from build123d import *

# Parameters (mm, degrees)
SKETCH1_R           = 1.5
BOSS_EXTRUDE1_DEPTH = 2
FILLET1_R           = 2


with BuildPart() as part:
    # Sketch1 → Boss-Extrude1 (new body)
    with BuildSketch(Plane(origin=(0, 0, 0), x_dir=(1, 0, 0), z_dir=(0, 1, 0))):
        Polygon((-18, 18), (18, 18), (18, -18), (8, -18), (8, -34), (-8, -34), (-8, -18), (-18, -18), align=None)
        with Locations(Location((-15, 15, 0), (0, 0, 270))):
            Circle(SKETCH1_R, mode=Mode.SUBTRACT)
        with Locations(Location((15, 15, 0), (0, 0, 90))):
            Circle(SKETCH1_R, mode=Mode.SUBTRACT)
        with Locations(Location((15, -15, 0), (0, 0, 270))):
            Circle(SKETCH1_R, mode=Mode.SUBTRACT)
        with Locations(Location((-15, -15, 0), (0, 0, 90))):
            Circle(SKETCH1_R, mode=Mode.SUBTRACT)
    extrude(amount=BOSS_EXTRUDE1_DEPTH)

    # Fillet1
    fillet1_edges = [part.edges().sort_by_distance(p)[0] for p in [
        (8, 1, 18),
        (8, 1, 34),
        (-8, 1, 34),
        (-8, 1, 18),
        (-18, 1, 18),
        (-18, 1, -18),
        (18, 1, -18),
        (18, 1, 18),
    ]]
    fillet(fillet1_edges, radius=FILLET1_R)


solid = part.part
The model under review builds one solid part; all positions refer to its coordinate system, in mm. A direction names the side the tool comes from. Coordinates: 2 decimals unless noted, no trailing zeros. Loops run counter-clockwise (first coordinate to the right, second up) from the corner with the lowest first, then second, coordinate; pieces in that order, holes last. Notation, with made-up numbers: (-12, 45) -> (7, 45) arc R23 cw to (7, 54) -> close; hole circle Ø4 at (37.25, 88.5). An arc over 180 degrees is marked (long way). Use a Markdown table: item, result. Add a question column.
1. Machinability: for faces 1 (the face through (-8, 1, 26)), 2 (the face through (14.93, 0.99, -13.5)), 3 (the face through (8, 1, 26)), which of the approach directions +Z, -Z, +X, -X, +Y, -Y give a long, thin tool a straight path to every point of the face, cutting with its end or side? Answer none if there is none.
2. Add section D-D on z = 24. Write out the cut boundary in (x, y), plus the area to 3 significant figures.
3. Add section A-A on z = -15. Write out the cut boundary in (x, y), plus the area to 3 significant figures.
4. Add section C-C on y = 1.55. Write out the cut boundary in (x, z), plus the area to 3 significant figures.
5. Add section B-B on x = -15. Write out the cut boundary in (y, z).
6. To check wall thickness, follow line 1 (X direction, y = 1, z = -15); line 2 (Z direction, x = 15.5, y = 1.8); line 3 (X direction, y = 0.4, z = 31.5). State the ranges of each line that lie inside material, in increasing order.
7. Draft analysis for pull direction Z (two halves, no side actions). For faces 4 (the face through (13, 1, 18)), 5 (the face through (15.07, 0.99, 13.5)), 6 (the face through (0, 0, 2)), state which applies: pulls with the +Z half, pulls with the -Z half, needs draft (parallel to the pull), parting line crosses it, or undercut.
8. Clearance check with flat-ended pins moving along their axes: pin 1 Ø0.6 at (y, z) = (1.5, 29) entering from -X; pin 2 Ø2.5 at (x, z) = (15, -15) entering from -Y; pin 3 Ø1 at (y, z) = (1.5, 26) entering from +X. State where each tip first meets the part, or that it passes through.
Returned:
| question | item | result |
|---|---|---|
| 1 | face 1 | +Z, -X, +Y, -Y |
| 1 | face 2 | +Y, -Y |
| 1 | face 3 | +Z, +X, +Y, -Y |
| 2 | outline | (-8, 0) -> (8, 0) -> (8, 2) -> (-8, 2) -> close |
| 2 | area | 32.0 mm² |
| 3 | outline | (-18, 0) -> (-16.5, 0) -> (-16.5, 2) -> (-18, 2) -> close; (-13.5, 0) -> (13.5, 0) -> (13.5, 2) -> (-13.5, 2) -> close; (16.5, 0) -> (18, 0) -> (18, 2) -> (16.5, 2) -> close |
| 3 | area | 60.0 mm² |
| 4 | outline | (-18, -16) arc R2 ccw to (-16, -18) -> (16, -18) arc R2 ccw to (18, -16) -> (18, 16) arc R2 ccw to (16, 18) -> (10, 18) arc R2 cw to (8, 20) -> (8, 32) arc R2 ccw to (6, 34) -> (-6, 34) arc R2 ccw to (-8, 32) -> (-8, 20) arc R2 cw to (-10, 18) -> (-16, 18) arc R2 ccw to (-18, 16) -> close; hole circle Ø3 at (-15, -15); hole circle Ø3 at (-15, 15); hole circle Ø3 at (15, -15); hole circle Ø3 at (15, 15) |
| 4 | area | 1,520 mm² |
| 5 | outline | (0, -18) -> (2, -18) -> (2, -16.5) -> (0, -16.5) -> close; (0, -13.5) -> (2, -13.5) -> (2, 13.5) -> (0, 13.5) -> close; (0, 16.5) -> (2, 16.5) -> (2, 18) -> (0, 18) -> close |
| 6 | line 1 | x = -18 to -16.5, -13.5 to 13.5, 16.5 to 18 |
| 6 | line 2 | z = -18 to -16.41, -13.59 to 13.59, 16.41 to 18 |
| 6 | line 3 | x = -8 to 8 |
| 7 | face 4 | pulls with the +Z half |
| 7 | face 5 | undercut |
| 7 | face 6 | needs draft |
| 8 | pin 1 | stops at x = -8 |
| 8 | pin 2 | passes through |
| 8 | pin 3 | stops at x = 8 |
